For this review, take the finished solid that the model builds, in its own axes (mm). A direction names the side the tool comes from. Give positions to 0.01 mm unless a question says otherwise; leave off trailing zeros. Write each loop counter-clockwise with the first axis right and the second up, starting at its lowest first coordinate (ties: lowest second). Pieces come first, ordered by that corner, then holes. Notation, with made-up numbers: (54.25, 34.25) -> (78.25, 34.25) arc R15 cw to (78.25, 41.25) -> close; hole circle Ø10 at (49.25, -37). An arc over 180 degrees is marked (long way). Write item = value, one per line.
```python
from build123d import *

# Parameters (mm, degrees)
CROQUIS3_R              = 3.175
SALIENTE_EXTRUIR2_DEPTH = 1.5875
SALIENTE_EXTRUIR3_DEPTH = 25


with BuildPart() as part:
    # Croquis3 → Saliente-Extruir2 (new body)
    with BuildSketch(Plane.XY):
        Polygon((0, -17), (0, 0), (-30, 0), (-30, -12), align=None)
        with Locations((-25, -5)):
            Circle(CROQUIS3_R, mode=Mode.SUBTRACT)
        with Locations((-5, -5)):
            Circle(CROQUIS3_R, mode=Mode.SUBTRACT)
    extrude(amount=SALIENTE_EXTRUIR2_DEPTH)

    # Croquis4 → Saliente-Extruir3 (add)
    with BuildSketch(Plane.XY.offset(1.5875)):
        Polygon((-30, -12), (0, -17), (0, -15.390602414), (-30, -10.390602414), align=None)
    extrude(amount=SALIENTE_EXTRUIR3_DEPTH)


solid = part.part
```
(1) Tool access review of faces 5 (the face through (-14.79, -12.926, 13.912)), 6 (the face through (-30, -11, 10)): name each direction out of +Z, -Z, +X, -X, +Y, -Y from which nothing blocks a thin tool from reaching the whole face with its end or side.
Answers below:
face_5 = +Z, +X, +Y
face_6 = +Z, -Z, -X, +Y, -Y
(2) Take a section at D-D (x = -5). Write out the cut boundary in (y, z) (1 decimal), plus the area to 3 significant figures.
Answers below:
outline = (-16.2, 0) -> (-8.2, 0) -> (-8.2, 1.6) -> (-14.6, 1.6) -> (-14.6, 26.6) -> (-16.2, 26.6) -> close; (-1.8, 0) -> (0, 0) -> (0, 1.6) -> (-1.8, 1.6) -> close
area = 55.8 mm^2
(3) Take a section at C-C (z = 11.5). Write out the cut boundary in (x, y), plus the area to 3 significant figures.
Answers below:
outline = (-30, -12) -> (0, -17) -> (0, -15.39) -> (-30, -10.39) -> close
area = 48.3 mm^2
(4) The part is to be moulded in two halves that separate along Y. For faces 1 (the face through (-15, 0, 1)), 2 (the face through (-15.21, -14.465, 13.108)), 3 (the face through (-28.17, -4.86, 0.78)), 4 (the face through (0, -16, 9)), say which applies: released by +Y, released by -Y, zero draft, split by the parting line, or undercut.
Answers below:
face_1 = released by +Y
face_2 = released by -Y
face_3 = undercut
face_4 = zero draft
(5) To check wall thickness, follow probe 1 along X at (y, z) = (-4.75, 1.25); probe 2 along Z at (x, y) = (-8.25, -9); probe 3 along Y at (x, z) = (-4, 1). State the ranges of each line that lie inside material, in increasing order.
Answers below:
probe_1 = -30 to -28.17, -21.83 to -8.17, -1.83 to 0
probe_2 = 0 to 1.59
probe_3 = -16.33 to -8.01, -1.99 to 0
(6) Take a section at A-A (x = -25). Write out the cut boundary in (y, z) (1 decimal), plus the area to 3 significant figures.
Answers below:
outline = (-12.8, 0) -> (-8.2, 0) -> (-8.2, 1.6) -> (-11.2, 1.6) -> (-11.2, 26.6) -> (-12.8, 26.6) -> close; (-1.8, 0) -> (0, 0) -> (0, 1.6) -> (-1.8, 1.6) -> close
area = 50.5 mm^2
(7) Take a section at B-B (y = -5). Write out the cut boundary in (x, z) (1 decimal), plus the area to 3 significant figures.
Answers below:
outline = (-30, 0) -> (-28.2, 0) -> (-28.2, 1.6) -> (-30, 1.6) -> close; (-21.8, 0) -> (-8.2, 0) -> (-8.2, 1.6) -> (-21.8, 1.6) -> close; (-1.8, 0) -> (0, 0) -> (0, 1.6) -> (-1.8, 1.6) -> close
area = 27.5 mm^2
